```python
from build123d import *

# Parameters (mm, degrees)
SKETCH_W      = 126.7
SKETCH_H      = 76.5
PAD_DEPTH     = 7
SKETCH001_R   = 2
SKETCH001_R_2 = 3
POCKET_DEPTH  = 50


with BuildPart() as pocket:
    # Sketch → Pad (new body)
    with BuildSketch(Plane.XY):
        with Locations((63.35, 38.25)):
            Rectangle(SKETCH_W, SKETCH_H)
    extrude(amount=PAD_DEPTH)

    # Sketch001 → Pocket (cut)
    with BuildSketch(Plane.XY.offset(7)):
        with Locations((0, 66.2)):
            Circle(SKETCH001_R)
        with Locations((70, 8)):
            Circle(SKETCH001_R)
        with Locations((118.7, 66.2)):
            Circle(SKETCH001_R_2)
        with Locations((118.7, 10)):
            Circle(SKETCH001_R_2)
        with Locations((45, 19)):
            Circle(SKETCH001_R_2)
    extrude(amount=-POCKET_DEPTH, mode=Mode.SUBTRACT)


with BuildPart() as fusion:
    # Part__Mirroring: instance of Pocket
    add(pocket.part.mirror(Plane(origin=(0, 0, 0), x_dir=(0, -1, 0), z_dir=(1, 0, 0))))

    # Fusion: union Pocket
    add(pocket.part)


solid = fusion.part
```
The listing builds one solid part. Answer for the finished solid, in the listing's coordinates (mm). Give positions to 0.01 mm unless a question says otherwise; leave off trailing zeros. Order: outer loops, then holes, each group sorted by start corner. A loop starts at its lowest first (then second) coordinate and runs counter-clockwise, first axis right, second up. Notation, with made-up numbers: (-37, 11.5) -> (7, 11.5) arc R29 cw to (7, 42.5) -> close; hole circle Ø6 at (-19, 37). An arc over 180 degrees is marked (long way). Answer as a JSON object with one key per item and string values. Group by question number.
Item 1: The part is cut by section B-B on x = -45. Write down the section's boundary in (y, z), and give its area (4 significant figures).
Item 2: The part is cut by section A-A on x = 118.7. Write down the section's boundary in (y, z).
Item 3: A flat-ended cylindrical pin translates along its axis: pin 1 (5.5 mm diameter, centred on x = -118.7, y = 66.2, fed in from -Z). Find the tip coordinate at first contact, or state that the pin passes through.
Item 4: Consider L1, parallel to Y at x = 118.7, z = 5.75; L2, parallel to Y at x = 0, z = 3; L3, parallel to Y at x = 45, z = 3.5. Determine where each line is inside the solid, lowest interval first. Write a range as from..to.
Item 5: Determine the mould class of faces 1 (the flat face through (-126.7, 38, 3)), 2 (the flat face through (-2, 76.5, 3)), 3 (the cylindrical face through (42, 19, 4)) for opening direction X: pulls with the +X half, pulls with the -X half, needs draft (parallel to the pull), parting line crosses it, or undercut.
Item 6: The part is cut by section C-C on y = 19. Write down the section's boundary in (x, z), and give its area (3 significant figures).
Result set:
{
 "1": {"outline": "(0, 0) -> (16, 0) -> (16, 7) -> (0, 7) -> close; (22, 0) -> (76.5, 0) -> (76.5, 7) -> (22, 7) -> close", "area": "493.5 mm²"},
 "2": {"outline": "(0, 0) -> (7, 0) -> (7, 7) -> (0, 7) -> close; (13, 0) -> (63.2, 0) -> (63.2, 7) -> (13, 7) -> close; (69.2, 0) -> (76.5, 0) -> (76.5, 7) -> (69.2, 7) -> close"},
 "3": {"pin 1": "through"},
 "4": {"L1": "0..7, 13..63.2, 69.2..76.5", "L2": "0..64.2, 68.2..76.5", "L3": "0..16, 22..76.5"},
 "5": {"face 1": "pulls with the -X half", "face 2": "needs draft", "face 3": "undercut"},
 "6": {"outline": "(-126.7, 0) -> (-48, 0) -> (-48, 7) -> (-126.7, 7) -> close; (-42, 0) -> (42, 0) -> (42, 7) -> (-42, 7) -> close; (48, 0) -> (126.7, 0) -> (126.7, 7) -> (48, 7) -> close", "area": "1,690 mm²"}
}
